```python
from build123d import *

# Parameters (mm, degrees)
SKETCH_1_W          = 20.5
SKETCH_1_H          = 98.14
SKETCH_1_R          = 1.7
EXTRUDE_1_DEPTH     = 3
FILLET_1_R          = 5
EXTRUDE_2_DEPTH     = 3
FILLET_2_R          = 10
SKETCH_3_W          = 15
SKETCH_3_H          = 3
EXTRUDE_3_DEPTH     = 3
CUT_EXTRUDE_1_DEPTH = 10
CUT_EXTRUDE_2_DEPTH = 10
FILLET_3_R          = 5
FILLET_4_R          = 3
CUT_EXTRUDE_3_DEPTH = 10


with BuildPart() as part:
    # 草图1 → 凸台-拉伸1 (new body)
    with BuildSketch(Plane(origin=(0, 0, 0), x_dir=(1, 0, 0), z_dir=(0, 1, 0))):
        Rectangle(SKETCH_1_W, SKETCH_1_H)
        with Locations(Location((-5.135, 44.07, 0), (0, 0, 270))):
            Circle(SKETCH_1_R, mode=Mode.SUBTRACT)
        with Locations(Location((5.135, 44.07, 0), (0, 0, 270))):
            Circle(SKETCH_1_R, mode=Mode.SUBTRACT)
    extrude(amount=EXTRUDE_1_DEPTH)

    # 圆角1
    fillet_1_edges = [part.edges().sort_by_distance(p)[0] for p in [
        (-10.25, 1.5, -49.07),
        (10.25, 1.5, -49.07),
    ]]
    fillet(fillet_1_edges, radius=FILLET_1_R)

    # 草图2 → 凸台-拉伸2 (add)
    with BuildSketch(Plane(origin=(0, 3, 0), x_dir=(1, 0, 0), z_dir=(0, 1, 0))):
        Polygon((-10.25, 30.93), (-25.25, -49.07), (-10.25, -49.07), align=None)
        Polygon((10.25, 30.93), (10.25, -49.07), (25.25, -49.07), align=None)
    extrude(amount=-EXTRUDE_2_DEPTH)

    # 圆角2
    fillet_2_edges = [part.edges().sort_by_distance(p)[0] for p in [
        (-10.25, 1.5, -30.93),
        (10.25, 1.5, -30.93),
    ]]
    fillet(fillet_2_edges, radius=FILLET_2_R)

    # 草图3 → 凸台-拉伸3 (add)
    with BuildSketch(Plane(origin=(0, 3, 0), x_dir=(1, 0, 0), z_dir=(0, 1, 0))):
        with Locations((0, -50.57)):
            Rectangle(SKETCH_3_W, SKETCH_3_H)
    extrude(amount=-EXTRUDE_3_DEPTH)

    # 草图5 → 切除-拉伸1 (cut)
    with BuildSketch(Plane(origin=(0, 3, 0), x_dir=(1, 0, 0), z_dir=(0, 1, 0))):
        Polygon((-16.9, -49.07), (-16.9, -44.07), (-18.6, -44.07), (-18.6, -41.07), (-16.9, -41.07), (-16.9, -36.07), (-13.5, -36.07), (-13.5, -41.07), (-11.8, -41.07), (-11.8, -44.07), (-13.5, -44.07), (-13.5, -49.07), align=None)
        Polygon((13.5, -49.07), (16.9, -49.07), (16.9, -44.07), (18.6, -44.07), (18.6, -41.07), (16.9, -41.07), (16.9, -36.07), (13.5, -36.07), (13.5, -41.07), (11.8, -41.07), (11.8, -44.07), (13.5, -44.07), align=None)
    extrude(amount=-CUT_EXTRUDE_1_DEPTH, mode=Mode.SUBTRACT)

    # 草图6 → 切除-拉伸2 (cut)
    with BuildSketch(Plane(origin=(0, 3, 0), x_dir=(1, 0, 0), z_dir=(0, 1, 0))):
        Polygon((-2.459339702, 29.07), (2.459339702, 29.07), (13.148083743, -27.936634883), (0, -41.084718626), (-13.148083743, -27.936634883), align=None)
    extrude(amount=-CUT_EXTRUDE_2_DEPTH, mode=Mode.SUBTRACT)

    # 圆角3
    fillet_3_edges = [part.edges().sort_by_distance(p)[0] for p in [
        (-13.148083743, 1.5, 27.936634883),
        (13.148083743, 1.5, 27.936634883),
        (0, 1.5, 41.084718626),
    ]]
    fillet(fillet_3_edges, radius=FILLET_3_R)

    # 圆角4
    fillet_4_edges = [part.edges().sort_by_distance(p)[0] for p in [
        (-25.25, 1.5, 49.07),
        (25.25, 1.5, 49.07),
    ]]
    fillet(fillet_4_edges, radius=FILLET_4_R)

    # 草图7 → 切除-拉伸3 (cut)
    with BuildSketch(Plane.XZ):
        with BuildLine():
            Line((-18.6, 44.07), (-18.6, 41.07))
            ThreePointArc((-18.6, 41.07), (-20.756776436, 42.57), (-18.6, 44.07))
        make_face()
        with BuildLine():
            Line((-11.8, 44.07), (-11.8, 41.07))
            ThreePointArc((-11.8, 41.07), (-9.643223564, 42.57), (-11.8, 44.07))
        make_face()
        with BuildLine():
            Line((11.8, 44.07), (11.8, 41.07))
            ThreePointArc((11.8, 41.07), (9.643223564, 42.57), (11.8, 44.07))
        make_face()
        with BuildLine():
            Line((18.6, 44.07), (18.6, 41.07))
            ThreePointArc((18.6, 41.07), (20.756776436, 42.57), (18.6, 44.07))
        make_face()
    extrude(amount=-CUT_EXTRUDE_3_DEPTH, mode=Mode.SUBTRACT)


solid = part.part
```
Model file for the job. Use its own axes, mm. A direction names the side the tool comes from. Coordinates: 2 decimals unless noted, no trailing zeros. Loops run counter-clockwise (first coordinate to the right, second up) from the corner with the lowest first, then second, coordinate; pieces in that order, holes last. Notation, with made-up numbers: M 59.5,80.25 L 89.5,80.25 A4 ccw 89.5,85.25 Z; hole C -25,13.5 d6. An arc over 180 degrees is marked long. Use CSV: the item, a comma, the result in double quotes. Start each with the question number.
1. Band-saw the part on A-A, the plane z = -4.5. List the corners of the cut face in (x, y), then the cut area to 3 significant figures.
2. Two-plate mould, pull along X, no slides. Class faces 1 (the cylindrical face through (8.75, 1.52, -47.64)), 2 (the flat face through (10, 2, 49.07)), 3 (the flat face through (-17.4, 1.5, 7.2)), 4 (the flat face through (16.9, 2, 47)): pulls with the +X half, pulls with the -X half, needs draft (parallel to the pull), parting line crosses it, or undercut.
3. Probe probe 1 along X at (y, z) = (1.9, -44.07) (3 decimals); probe 2 along X at (y, z) = (2.15, -33.5); probe 3 along X at (y, z) = (1.75, 42.57). List the from-to ranges inside material, lowest first. Write a range as [from, to].
4. Band-saw the part on C-C, the plane x = -15.5. List the corners of the cut face in (y, z), then the cut area to 3 significant figures.
5. Band-saw the part on D-D, the plane z = -33. List the corners of the cut face in (x, y).
6. Band-saw the part on B-B, the plane z = 42.57. List the corners of the cut face in (x, y).
7. Tool access for faces 5 (the flat face through (0, 2, -29.07)), 6 (the flat face through (-16.9, 2, 47)), 7 (the flat face through (-7.5, 2, 51)): list every direction of +Z, -Z, +X, -X, +Y, -Y with a clear straight run to the whole face (end or side of a thin tool).
8. Flat gauge pin, fed straight in: pin 1 (1.5 mm diameter, centred on x = -19, y = 1.5, fed in from +Z). Where does the tip first touch, or does it go through?
Entries:
1,outline,"M -15.21,0 L -7.07,0 L -7.07,3 L -15.21,3 Z; M 7.07,0 L 15.21,0 L 15.21,3 L 7.07,3 Z"
1,area,"48.8 mm2"
2,face 1,"pulls with the +X half"
2,face 2,"needs draft"
2,face 3,"pulls with the -X half"
2,face 4,"undercut"
3,probe 1,"x = [-10.25, -6.835], [-3.435, 3.435], [6.835, 10.25]"
3,probe 2,"x = [-10.25, 10.25]"
3,probe 3,"x = [-24.03, -20.76], [-9.64, 9.64], [20.76, 24.03]"
4,outline,"M 0,-2.93 L 3,-2.93 L 3,36.07 L 0,36.07 Z"
4,area,"117 mm2"
5,outline,"M -10.25,0 L 10.25,0 L 10.25,3 L -10.25,3 Z"
6,outline,"M -24.03,0 L -20.76,0 L -20.76,3 L -24.03,3 Z; M -9.64,0 L 9.64,0 L 9.64,3 L -9.64,3 Z; M 20.76,0 L 24.03,0 L 24.03,3 L 20.76,3 Z"
7,face 5,"+Y, -Y"
7,face 6,"+Z, +Y, -Y"
7,face 7,"+Z, -X, +Y, -Y"
8,pin 1,"stops at z = 49.07"
